The listing builds one solid part. Answer for the finished solid, in the listing's coordinates (mm). Face numbers are marked on the shaded views. A direction names the side the tool comes from. Give positions to 0.01 mm unless a question says otherwise; leave off trailing zeros. Write each loop counter-clockwise with the first axis right and the second up, starting at its lowest first coordinate (ties: lowest second). Pieces come first, ordered by that corner, then holes. Notation, with made-up numbers: (88.5, 22.25) - (119.5, 22.25) arc R23 ccw to (119.5, 57.25) - close; hole circle Ø5 at (-14, 22). An arc over 180 degrees is marked (long way). Return JSON: item names as keys, results as strings.
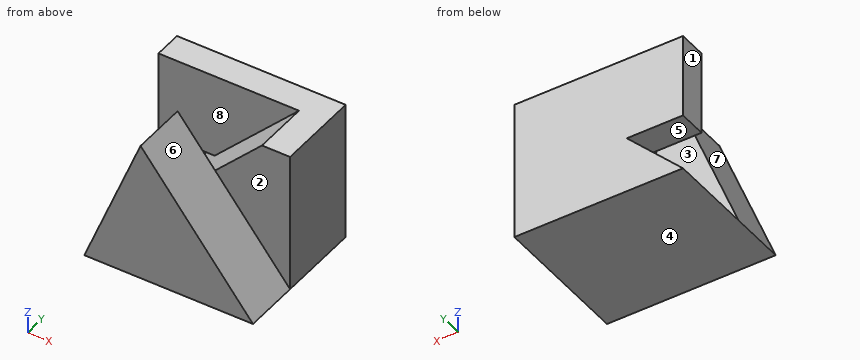
from build123d import *

# Parameters (mm, degrees)
SKETCH3_W           = 6
SKETCH3_H           = 5
BOSS_EXTRUDE1_DEPTH = 5
CUT_EXTRUDE1_DEPTH  = 3
CUT_EXTRUDE2_DEPTH  = 3
SKETCH6_W           = 3
SKETCH6_H           = 1
BOSS_EXTRUDE2_DEPTH = 6
CUT_EXTRUDE3_DEPTH  = 2


with BuildPart() as part:
    # Sketch3 → Boss-Extrude1 (new body)
    with BuildSketch(Plane.XY):
        with Locations((3, 2.5)):
            Rectangle(SKETCH3_W, SKETCH3_H)
    extrude(amount=BOSS_EXTRUDE1_DEPTH)

    # Sketch4 → Cut-Extrude1 (cut)
    with BuildSketch(Plane(origin=(0, 5, 0), x_dir=(1, 0, 0), z_dir=(0, 1, 0))):
        Polygon((0, 0), (5, -5), (0, -5), align=None)
    extrude(amount=-CUT_EXTRUDE1_DEPTH, mode=Mode.SUBTRACT)

    # Sketch5 → Cut-Extrude2 (cut)
    with BuildSketch(Plane(origin=(0, 2, 0), x_dir=(1, 0, 0), z_dir=(0, 1, 0))):
        Polygon((0, 0), (2, -5), (0, -5), align=None)
    extrude(amount=-CUT_EXTRUDE2_DEPTH, mode=Mode.SUBTRACT)

    # Sketch6 → Boss-Extrude2 (add)
    with BuildSketch(Plane(origin=(6, 0, 0), x_dir=(0, 0, -1), z_dir=(1, 0, 0))):
        with Locations((-3.5, 4.5)):
            Rectangle(SKETCH6_W, SKETCH6_H)
    extrude(amount=-BOSS_EXTRUDE2_DEPTH)

    # Sketch7 → Cut-Extrude3 (cut)
    with BuildSketch(Plane.XZ):
        Polygon((2, 5), (6, 0), (6, 5), align=None)
    extrude(amount=-CUT_EXTRUDE3_DEPTH, mode=Mode.SUBTRACT)


solid = part.part
Item 1: For the marked faces 4, 5, 6, 7 and 8, determine the directions among +Z, -Z, +X, -X, +Y, -Y from which every point of the face is accessible in a straight line to the end or side of a thin tool.
Answer below:
{"face 4": "-Z, +X, -X, +Y, -Y", "face 5": "-X, +Y", "face 6": "+Z, +X, -Y", "face 7": "+Z, -X, -Y", "face 8": "+Z, -X"}
Item 2: The mould has two halves that part along Y. Classify the marked faces 1, 2 and 3: +Y half, -Y half, draft (parallel to the pull), parting line (faces both ways), or undercut.
Answer below:
{"face 1": "draft", "face 2": "-Y half", "face 3": "undercut"}
Item 3: A flat-ended cylindrical pin translates along its axis: P1, Ø2, axis at x = 0.5, z = 3.5, coming from the -Y side. Find the tip coordinate at first contact, or state that the pin passes through.
Answer below:
{"P1": "stops at y = 0"}
Item 4: A cutting plane is placed at D-D on z = 3.1. Determine the outline of the cut face in (x, y), then the cut area to 3 significant figures.
Answer below:
{"outline": "(0, 4) - (3.1, 4) - (3.1, 2) - (1.24, 2) - (1.24, 0) - (3.52, 0) - (3.52, 2) - (6, 2) - (6, 5) - (0, 5) - close", "area": "16.4 mm²"}
Item 5: Consider L1, parallel to Y at x = 2.1, z = 2.75; L2, parallel to Y at x = 5.75, z = 3.2; L3, parallel to Y at x = 3.85, z = 4.85. Determine where each line is inside the solid, lowest interval first.
Answer below:
{"L1": "y = 0 to 2, 4 to 5", "L2": "y = 2 to 5", "L3": "y = 4 to 5"}
Item 6: A cutting plane is placed at C-C on x = 2.6. Determine the outline of the cut face in (y, z), then the cut area to 3 significant figures.
Answer below:
{"outline": "(0, 0) - (5, 0) - (5, 5) - (4, 5) - (4, 2.6) - (2, 2.6) - (2, 4.25) - (0, 4.25) - close", "area": "18.7 mm²"}
Item 7: A cutting plane is placed at B-B on x = 1. Determine the outline of the cut face in (y, z).
Answer below:
{"outline": "(0, 0) - (5, 0) - (5, 1) - (2, 1) - (2, 2.5) - (0, 2.5) - close; (4, 2) - (5, 2) - (5, 5) - (4, 5) - close"}
Item 8: A cutting plane is placed at A-A on z = 3.9. Determine the outline of the cut face in (x, y), then the cut area to 3 significant figures.
Answer below:
{"outline": "(0, 4) - (3.9, 4) - (3.9, 2) - (6, 2) - (6, 5) - (0, 5) - close; (1.56, 0) - (2.88, 0) - (2.88, 2) - (1.56, 2) - close", "area": "12.8 mm²"}
